Work out the finished part from the listing and answer in its coordinate system (mm). Face numbers are marked on the shaded views. A direction names the side the tool comes from. Coordinates: 2 decimals unless noted, no trailing zeros. Write each loop counter-clockwise with the first axis right and the second up, starting at its lowest first coordinate (ties: lowest second). Pieces come first, ordered by that corner, then holes. Notation, with made-up numbers: (47.25, 28.5) - (99.25, 28.5) arc R13 cw to (99.25, 49.5) - close; hole circle Ø11 at (-25.5, 21). An arc over 180 degrees is marked (long way). Answer as a JSON object with one key per item and string values. Group by question number.
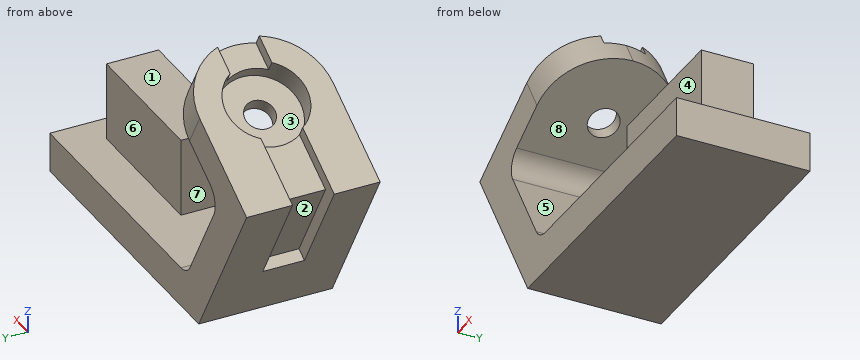
from build123d import *

# Parameters (mm, degrees)
F1_DEPTH  = 64
F3_DEPTH  = 25
F4_R      = 19.5
F4_R_2    = 6
F5_DEPTH  = 12
F6_R      = 7.2312800618
F7_DEPTH  = 7
F8_W      = 20
F8_H      = 56
F9_DEPTH  = 6
F10_W     = 88.7789055705
F10_H     = 20
F11_DEPTH = 6
F12_R     = 10
F13_R     = 10
F14_W     = 70
F14_H     = 25
F15_DEPTH = 37.5


with BuildPart() as f1:
    # F0 (on Front) → F1 (new body)
    with BuildSketch(Plane.XZ):
        Polygon((-45, 77.9422863406), (0, 0), (140, 0), (140, 19), (10.9696551146, 19), (-19.0455173281, 70.9878036687), (36.3801085141, 102.9878036687), (26.8801085141, 119.4422863406), align=None)
    extrude(amount=-F1_DEPTH)

    # F2 (on face) → F3 (cut)
    with BuildSketch(Plane(origin=(-45, 0, 77.9422863406), x_dir=(0.8660254038, 0, 0.5), z_dir=(-0.5, 0, 0.8660254038))):
        with BuildLine():
            ThreePointArc((51, 64), (73.627416998, 54.627416998), (83, 32))
            Line((83, 32), (83, 64))
            Line((83, 64), (51, 64))
        make_face()
        with BuildLine():
            Line((83, 0), (83, 32))
            ThreePointArc((83, 32), (73.627416998, 9.372583002), (51, 0))
            Line((51, 0), (83, 0))
        make_face()
    extrude(amount=-F3_DEPTH, mode=Mode.SUBTRACT)

    # F4 (on face) → F5 (cut)
    with BuildSketch(Plane(origin=(-45, 0, 77.9422863406), x_dir=(0.8660254038, 0, 0.5), z_dir=(-0.5, 0, 0.8660254038))):
        with Locations((51, 32)):
            Circle(F4_R)
        with Locations((51, 32)):
            Circle(F4_R_2, mode=Mode.SUBTRACT)
        with Locations((51, 32)):
            Circle(F4_R_2)
    extrude(amount=-F5_DEPTH, mode=Mode.SUBTRACT)

    # F6 (on face) → F7 (cut, through all)
    with BuildSketch(Plane(origin=(-39, 0, 67.5499814952), x_dir=(0.8660254038, 0, 0.5), z_dir=(-0.5, 0, 0.8660254038))):
        with Locations((51, 32)):
            Circle(F6_R)
    extrude(amount=-F7_DEPTH, mode=Mode.SUBTRACT)

    # F8 (on face) → F9 (cut)
    with BuildSketch(Plane(origin=(0, 0, 0), x_dir=(0, -1, 0), z_dir=(-0.8660254038, 0, -0.5))):
        with Locations((-32, 62)):
            Rectangle(F8_W, F8_H)
    extrude(amount=-F9_DEPTH, mode=Mode.SUBTRACT)

    # F10 (on face) → F11 (cut)
    with BuildSketch(Plane(origin=(-45, 0, 77.9422863406), x_dir=(0.8660254038, 0, 0.5), z_dir=(-0.5, 0, 0.8660254038))):
        with Locations((44.3894527853, 32)):
            Rectangle(F10_W, F10_H)
    extrude(amount=-F11_DEPTH, mode=Mode.SUBTRACT)

    # F12
    f12_edges = [f1.edges().sort_by_distance(p)[0] for p in [
        (-19.045517, 32, 70.987804),
    ]]
    fillet(f12_edges, radius=F12_R)

    # F13
    f13_edges = [f1.edges().sort_by_distance(p)[0] for p in [
        (10.969655, 32, 19),
    ]]
    fillet(f13_edges, radius=F13_R)

    # F14 (on face) → F15 (join)
    with BuildSketch(Plane.XY.offset(19)):
        with Locations((90, 32)):
            Rectangle(F14_W, F14_H)
    extrude(amount=F15_DEPTH)


solid = f1.part
Q1. Section A-A on z = 53.5 is taken. Determine the outline of the cut face in (x, y).
Q2. Flat-ended cylindrical pins translate along their axes: pin 1 Ø12.5 at (x, y) = (78, 31.5) entering from +Z; pin 2 Ø19 at (x, z) = (105.5, 34) entering from -Y; pin 3 Ø6 at (y, z) = (35.5, 52.5) entering from +X. Find the tip coordinate at first contact, or state that the pin passes through.
Q3. Section C-C on y = 16.5 is taken. Determine the outline of the cut face in (x, z), plus the area to 3 significant figures.
Q4. Section D-D on z = 80 is taken. Determine the outline of the cut face in (x, y).
Q5. Section B-B on x = 75 is taken. Determine the outline of the cut face in (y, z).
Q6. For a pull along X with two mould halves and no side action, classify the marked faces 6, 7 and 8 as +X half, -X half, draft (parallel to the pull), parting line (faces both ways), or undercut.
Q7. A tool of negligible diameter and unlimited length cuts with its end or side. For the marked faces 1, 2, 3, 4 and 5, from which of +Z, -Z, +X, -X, +Y, -Y can it reach the whole face along a straight path? Write none if from no direction.
Q8. Consider L1, parallel to Z at x = -7.5, y = 18.5; L2, parallel to Z at x = 87, y = 3; L3, parallel to Y at x = 90, z = 40.5. Determine where each line is inside the solid, lowest interval first. Write a range as from..to.
Numbers:
{
 "1": {"outline": "(-30.89, 0) - (-8.95, 0) - (-8.95, 64) - (-30.89, 64) - (-30.89, 42) - (-23.96, 42) - (-23.96, 22) - (-30.89, 22) - close; (55, 19.5) - (125, 19.5) - (125, 44.5) - (55, 44.5) - close"},
 "2": {"pin 1": "stops at z = 56.5", "pin 2": "stops at y = 19.5", "pin 3": "stops at x = 125"},
 "3": {"outline": "(-45, 77.94) - (0, 0) - (140, 0) - (140, 19) - (16.74, 19) arc R10 cw to (8.08, 24) - (-14.05, 62.33) arc R10 cw to (-10.39, 75.99) - (32.91, 100.99) - (23.41, 117.44) - (9.41, 109.36) - (15.41, 98.97) - (-5.08, 87.13) - (-11.08, 97.53) - close", "area": "5,040 mm²"},
 "4": {"outline": "(-41.44, 0) - (-3.44, 0) - (-3.44, 64) - (-41.44, 64) - (-41.44, 42) - (-29.44, 42) - (-29.44, 22) - (-41.44, 22) - close"},
 "5": {"outline": "(0, 0) - (64, 0) - (64, 19) - (44.5, 19) - (44.5, 56.5) - (19.5, 56.5) - (19.5, 19) - (0, 19) - close"},
 "6": {"face 6": "draft", "face 7": "undercut", "face 8": "+X half"},
 "7": {"face 1": "+Z, +X, +Y, -Y", "face 2": "-X", "face 3": "none", "face 4": "+Z, +X, -Y", "face 5": "+Y, -Y"},
 "8": {"L1": "z = 12.99..50.99, 77.65..86.85", "L2": "z = 0..19", "L3": "y = 19.5..44.5"}
}
